Build history of the part. All positions in model axes, mm. A direction names the side the tool comes from. Coordinates: 2 decimals unless noted, no trailing zeros. Order: outer loops, then holes, each group sorted by start corner. A loop starts at its lowest first (then second) coordinate and runs counter-clockwise, first axis right, second up. Notation, with made-up numbers: (67.5, -36.75) - (93.5, -36.75) arc R20 ccw to (93.5, 2.25) - close; hole circle Ø8 at (14.5, -4.5). An arc over 180 degrees is marked (long way). Write each question's results on one line, items separated by ' | '. Start each with the question number.
from build123d import *

# Parameters (mm, degrees)
CROQUIS2_W              = 58
CROQUIS2_H              = 26
CROQUIS2_W_2            = 44
CROQUIS2_H_2            = 22
SALIENTE_EXTRUIR3_DEPTH = 20
CROQUIS4_R              = 1
CROQUIS4_W              = 2.5
CROQUIS4_H              = 6
CUT_EXTRUDE1_DEPTH      = 39.327535793
SKETCH1_W               = 51
SKETCH1_H               = 20
BOSS_EXTRUDE1_DEPTH     = 2.5
CROQUIS6_R              = 2.75
SALIENTE_EXTRUIR5_DEPTH = 3
BOSS_EXTRUDE2_START     = -3
SKETCH3_R               = 0.75
SKETCH3_R_2             = 4.75
BOSS_EXTRUDE2_DEPTH     = 3
BOSS_EXTRUDE3_DEPTH     = 25
FILLET1_R               = 2
SKETCH6_R               = 2.15
BOSS_EXTRUDE4_DEPTH     = 5
FILLET4_R               = 1
BOSS_EXTRUDE5_DEPTH     = 20
BOSS_EXTRUDE6_REACH     = 93.885
CUT_EXTRUDE2_DEPTH      = 84.971155352


with BuildPart() as part:
    # Croquis2 → Saliente-Extruir3 (new body)
    with BuildSketch(Plane(origin=(0, 0, 0), x_dir=(1, 0, 0), z_dir=(0, 1, 0))):
        with Locations((-1, 0)):
            Rectangle(CROQUIS2_W, CROQUIS2_H)
        Rectangle(CROQUIS2_W_2, CROQUIS2_H_2, mode=Mode.SUBTRACT)
    extrude(amount=SALIENTE_EXTRUIR3_DEPTH)

    # Croquis4 → Cut-Extrude1 (cut, through all)
    with BuildSketch(Plane(origin=(0, 20, 0), x_dir=(1, 0, 0), z_dir=(0, 1, 0))):
        with Locations(Location((-24.5, 5, 0), (0, 0, 270))):
            Circle(CROQUIS4_R)
        with Locations(Location((-24.5, -5, 0), (0, 0, 270))):
            Circle(CROQUIS4_R)
        with Locations(Location((24.5, -5, 0), (0, 0, 90))):
            Circle(CROQUIS4_R)
        with Locations(Location((24.5, 5, 0), (0, 0, 90))):
            Circle(CROQUIS4_R)
        with Locations((23.25, 0)):
            Rectangle(CROQUIS4_W, CROQUIS4_H)
    extrude(amount=-CUT_EXTRUDE1_DEPTH, mode=Mode.SUBTRACT)

    # Sketch1 → Boss-Extrude1 (add)
    with BuildSketch(Plane.ZY.offset(30)):
        with Locations((0, 10)):
            Rectangle(SKETCH1_W, SKETCH1_H)
    extrude(amount=-BOSS_EXTRUDE1_DEPTH)

    # Croquis6 → Saliente-Extruir5 (add)
    with BuildSketch(Plane.XY.offset(25.5)):
        with BuildLine():
            Line((-39.436967742, 0), (-30, 0))
            Line((-30, 0), (-30, 20))
            Line((-30, 20), (-27.5, 20))
            Line((-27.5, 20), (-51.509432429, 48.613327353))
            ThreePointArc((-51.509432429, 48.613327353), (-67.00658501, 49.969152521), (-68.362410178, 34.47199994))
            Line((-68.362410178, 34.47199994), (-39.436967742, 0))
        make_face()
        with Locations((-59.935921303, 41.542663647)):
            Circle(CROQUIS6_R, mode=Mode.SUBTRACT)
    extrude(amount=-SALIENTE_EXTRUIR5_DEPTH)

    # Sketch3 → Boss-Extrude2 (add)
    with BuildSketch(Plane(origin=(0, 0, -25.5), x_dir=(-1, 0, 0), z_dir=(0, 0, -1)).offset(BOSS_EXTRUDE2_START)):
        with BuildLine():
            Line((51.509432429, 48.613327353), (27.5, 20))
            Line((27.5, 20), (30, 20))
            Line((30, 20), (30, 0))
            Line((30, 0), (39.436967742, 0))
            Line((39.436967742, 0), (68.362410178, 34.47199994))
            ThreePointArc((68.362410178, 34.47199994), (67.00658501, 49.969152521), (51.509432429, 48.613327353))
        make_face()
        with Locations((66.935921303, 41.542663647)):
            Circle(SKETCH3_R, mode=Mode.SUBTRACT)
        with Locations((59.935921303, 34.542663647)):
            Circle(SKETCH3_R, mode=Mode.SUBTRACT)
        with Locations((59.935921303, 48.542663647)):
            Circle(SKETCH3_R, mode=Mode.SUBTRACT)
        with Locations((52.935921303, 41.542663647)):
            Circle(SKETCH3_R, mode=Mode.SUBTRACT)
        with Locations((59.935921303, 41.542663647)):
            Circle(SKETCH3_R_2, mode=Mode.SUBTRACT)
    extrude(amount=BOSS_EXTRUDE2_DEPTH)

    # Sketch5 → Boss-Extrude3 (add)
    with BuildSketch(Plane(origin=(22, 0, 0), x_dir=(0, 0, -1), z_dir=(1, 0, 0))):
        Polygon((-13, 0), (-13, -12), (13, -12), (13, 0), (11, 0), (11, -10), (-11, -10), (-11, 0), align=None)
    extrude(amount=-BOSS_EXTRUDE3_DEPTH)

    # Fillet1
    fillet1_edges = [part.edges().sort_by_distance(p)[0] for p in [
        (28, 10, -13),
        (28, 10, 13),
    ]]
    fillet(fillet1_edges, radius=FILLET1_R)

    # Sketch6 → Boss-Extrude4 (add)
    with BuildSketch(Plane.XZ.offset(12)):
        with Locations(Location((10, 0, 0), (0, 0, 270))):
            Circle(SKETCH6_R)
    extrude(amount=BOSS_EXTRUDE4_DEPTH)

    # Fillet4
    fillet4_edges = [part.edges().sort_by_distance(p)[0] for p in [
        (10, -12, 2.15),
    ]]
    fillet(fillet4_edges, radius=FILLET4_R)

    # Sketch8 → Boss-Extrude5 (add)
    with BuildSketch(Plane(origin=(0, 20, 0), x_dir=(1, 0, 0), z_dir=(0, 1, 0))):
        Polygon((-27.5, 25.5), (-27.5, 13), (-15, 13), align=None)
        Polygon((-27.5, -13), (-15, -13), (-27.5, -25.5), align=None)
    extrude(amount=-BOSS_EXTRUDE5_DEPTH)

    # Boss-Extrude6: up to this plane
    boss_extrude6_end = Plane(origin=(-6.289584913, -5.277588381, 22.5), z_dir=(0.76604444311898, 0.642787609686537, 0))
    # Sketch9 → Boss-Extrude6 (add, up to the surface)
    with BuildSketch(Plane.XZ, mode=Mode.PRIVATE) as boss_extrude6_sk1:
        Polygon((-39.436967742, 22.5), (-26.5, 9.563032258), (-26.5, 22.5), align=None)
    boss_extrude6_tool1 = split(extrude(boss_extrude6_sk1.sketch, amount=-BOSS_EXTRUDE6_REACH, mode=Mode.PRIVATE), bisect_by=boss_extrude6_end, keep=Keep.BOTH, mode=Mode.PRIVATE)
    add(boss_extrude6_tool1.solids().sort_by_distance((-30.812323, 0, 18.187677))[0])
    # Sketch9 → Boss-Extrude6 (add, up to the surface)
    with BuildSketch(Plane.XZ, mode=Mode.PRIVATE) as boss_extrude6_sk2:
        Polygon((-26.5, -9.563032258), (-26.5, -22.5), (-39.436967742, -22.5), align=None)
    boss_extrude6_tool2 = split(extrude(boss_extrude6_sk2.sketch, amount=-BOSS_EXTRUDE6_REACH, mode=Mode.PRIVATE), bisect_by=boss_extrude6_end, keep=Keep.BOTH, mode=Mode.PRIVATE)
    add(boss_extrude6_tool2.solids().sort_by_distance((-30.812323, 0, -18.187677))[0])

    # Sketch10 → Cut-Extrude2 (cut, through all)
    with BuildSketch(Plane(origin=(0, 20, 0), x_dir=(1, 0, 0), z_dir=(0, 1, 0))):
        Polygon((-30, 13.063032258), (-30, -13.063032258), (-27.5, -10.563032258), (-27.5, 10.563032258), align=None)
    extrude(amount=-CUT_EXTRUDE2_DEPTH, mode=Mode.SUBTRACT)


solid = part.part
Item 1: Slice it at A-A (z = 0). Write the cut outline in (x, y), then the cut area to 3 significant figures.
Item 2: Slice it at C-C (x = 10). Write the cut outline in (y, z), then the cut area to 3 significant figures.
Item 3: Slice it at B-B (y = 32). Write the cut outline in (x, z), then the cut area to 3 significant figures.
Item 4: Which spindle directions (+Z, -Z, +X, -X, +Y, -Y) get a long thin tool onto all of the face, cutting with end or side? Do faces 4 (the flat face through (-33.552, 13.071, -16.615)), 5 (the flat face through (-22, 10, 0)), 6 (the flat face through (-6, 20, 11.2)), 7 (the flat face through (-25, 0, 2)). Say none if no direction does.
Item 5: Flat gauge pins, fed straight in: P1, Ø1.2, axis at x = -24.5, z = 5, coming from the -Y side; P2, Ø5, axis at x = 23.5, z = -3.5, coming from the -Y side; P3, Ø3, axis at y = 10.5, z = -0.5, coming from the -X side; P4, Ø12, axis at y = 25.5, z = -10.5, coming from the -X side. Where does each tip first touch, or does it go through?
Item 6: Slice it at D-D (x = -32.5). Write the cut outline in (y, z), then the cut area to 3 significant figures.
Item 7: Probe probe 1 along X at (y, z) = (12, -5); probe 2 along Z at (x, y) = (-24, 5); probe 3 along Z at (x, y) = (-11, 9). List the from-to ranges inside material, lowest first.
Item 8: Pull direction X, two halves, no side cores. Call faces 1 (the flat face through (-33.552, 13.55, 16.615)), 2 (the cylindrical face through (-67.19, 49.81, -23.98)), 3 (the flat face through (0, 8, 11)): released by +X, released by -X, zero draft, split by the parting line, or undercut.
Resolved:
1) outline: (-27.5, 0) - (-22, 0) - (-22, 20) - (-27.5, 20) - close; (-3, -12) - (6.85, -12) arc R1 cw to (7.85, -13) - (7.85, -17) - (12.15, -17) - (12.15, -13) arc R1 cw to (13.15, -12) - (22, -12) - (22, -10) - (-3, -10) - close; (24.5, 0) - (28, 0) - (28, 20) - (24.5, 20) - close | area: 252 mm^2
2) outline: (-17, -2.15) - (-13, -2.15) arc R1 cw to (-12, -3.15) - (-12, -13) - (20, -13) - (20, -11) - (-10, -11) - (-10, 11) - (20, 11) - (20, 13) - (-12, 13) - (-12, 3.15) arc R1 cw to (-13, 2.15) - (-17, 2.15) - close | area: 194 mm^2
3) outline: (-66.29, -25.5) - (-37.57, -25.5) - (-37.57, -20.63) - (-39.44, -22.5) - (-66.29, -22.5) - close; (-66.29, 22.5) - (-39.44, 22.5) - (-37.57, 20.63) - (-37.57, 25.5) - (-66.29, 25.5) - close | area: 176 mm^2
4) face 4: -X, +Y, -Y | face 5: +Y, -Y | face 6: +Z, -Z, +X, +Y | face 7: +Z, -Z, -X, -Y
5) P1: through | P2: y = -12 | P3: x = -27.5 | P4: x = -33.44
6) outline: (0, -25.5) - (25.96, -25.5) - (25.96, -15.56) - (0, -15.56) - close; (0, 15.56) - (25.96, 15.56) - (25.96, 25.5) - (0, 25.5) - close | area: 516 mm^2
7) probe 1: -27.5 to -25.5, -23.5 to -22, 22 to 23.5, 25.5 to 28 | probe 2: -22 to -5.87, -4.13 to 4.13, 5.87 to 22 | probe 3: -13 to -11, 11 to 13
8) face 1: released by -X | face 2: split by the parting line | face 3: undercut
